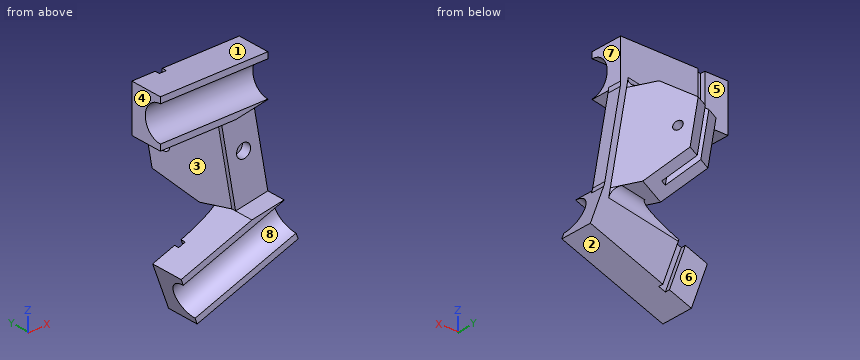
```python
from build123d import *

# Parameters (mm, degrees)
SKETCH2_W           = 58.42
SKETCH2_H           = 25.4
BOSS_EXTRUDE1_DEPTH = 17.78
CUT_EXTRUDE2_DEPTH  = 63.372388122
SKETCH6_W           = 3.81
SKETCH6_H           = 2.54
CUT_EXTRUDE3_DEPTH  = 25.4
CUT_EXTRUDE4_DEPTH  = 25.4
SKETCH8_W           = 17.78
SKETCH8_H           = 17.78
BOSS_EXTRUDE2_DEPTH = 25.4
SKETCH13_W          = 58.42
SKETCH13_H          = 9.398
CUT_EXTRUDE6_REACH  = 59.763
SKETCH15_W          = 25.4
SKETCH15_H          = 10.16
MIRROR14_START      = 9.31703521
MIRROR14_OUTLINE_W  = 7.62
MIRROR14_OUTLINE_H  = 25.4
MIRROR14_DEPTH      = 17.78
CUT_EXTRUDE7_DEPTH  = 25.4
BOSS_EXTRUDE3_DEPTH = 35.56
CUT_EXTRUDE8_REACH  = 128.018
CUT_EXTRUDE9_REACH  = 111.199
CUT_EXTRUDE10_REACH = 128.018
SKETCH25_R          = 2.4765
SKETCH26_R          = 3.81
CUT_EXTRUDE11_DEPTH = 5.08
FILLET1_R           = 15.24
FILLET2_R           = 5.08


with BuildPart() as part:
    # Sketch2 → Boss-Extrude1 (new body)
    with BuildSketch(Plane(origin=(0, 0, 0), x_dir=(1, 0, 0), z_dir=(0, 1, 0))):
        Rectangle(SKETCH2_W, SKETCH2_H)
    boss_extrude1 = extrude(amount=BOSS_EXTRUDE1_DEPTH)

    # Sketch4 → Cut-Extrude2 (cut, symmetric)
    with BuildSketch(Plane.ZY.offset(29.21)):
        with BuildLine():
            Line((-9.398, -66.725655712), (-9.398, 0))
            ThreePointArc((-9.398, 0), (0, 9.398), (9.398, 0))
            Line((9.398, 0), (9.398, -66.725655712))
            Line((9.398, -66.725655712), (9.398, -200.176967137))
            Line((9.398, -200.176967137), (-9.398, -200.176967137))
            Line((-9.398, -200.176967137), (-9.398, -66.725655712))
        make_face()
    cut_extrude2 = extrude(amount=CUT_EXTRUDE2_DEPTH, both=True, mode=Mode.SUBTRACT)

    # Sketch6 → Cut-Extrude3 (cut)
    with BuildSketch(Plane(origin=(0, 0, -12.7), x_dir=(-1, 0, 0), z_dir=(0, 0, -1))):
        with Locations((14.605, 16.51)):
            Rectangle(SKETCH6_W, SKETCH6_H)
    cut_extrude3 = extrude(amount=-CUT_EXTRUDE3_DEPTH, mode=Mode.SUBTRACT)

    # Sketch7 → Cut-Extrude4 (cut)
    with BuildSketch(Plane(origin=(0, 17.78, 0), x_dir=(1, 0, 0), z_dir=(0, 1, 0))):
        Polygon((11.700118151, 12.7), (29.21, 9.612535401), (29.21, 12.7), align=None)
    extrude(amount=-CUT_EXTRUDE4_DEPTH, mode=Mode.SUBTRACT)

    # Sketch8 → Boss-Extrude2 (add)
    with BuildSketch(Plane(origin=(2.524629641, 0, -14.317886186), x_dir=(-0.9848077530122094, 0, -0.17364817766692317), z_dir=(0.17364817766692317, 0, -0.9848077530122094))):
        with Locations((-18.20703521, 8.89)):
            Rectangle(SKETCH8_W, SKETCH8_H)
    extrude(amount=BOSS_EXTRUDE2_DEPTH)

    # Sketch13 → Cut-Revolve2 (revolve, cut)
    with BuildSketch(Plane.XZ):
        with Locations((0, 4.699)):
            Rectangle(SKETCH13_W, SKETCH13_H)
    revolve(axis=Axis((28.421300087, 0, 0), (-1, 0, 0)), mode=Mode.SUBTRACT)

    # Sketch15 → Cut-Extrude6 (cut, up to next)
    with BuildSketch(Plane(origin=(9.17548851, 0, 1.617886186), x_dir=(-0.17364817766692317, 0, 0.9848077530122095), z_dir=(-0.9848077530122095, 0, -0.17364817766692317)), mode=Mode.PRIVATE) as cut_extrude6_sk1:
        with Locations((-27.238762659, 5.08)):
            Rectangle(SKETCH15_W, SKETCH15_H)
    cut_extrude6_tool1 = extrude(cut_extrude6_sk1.sketch, amount=-CUT_EXTRUDE6_REACH, mode=Mode.PRIVATE) & part.part
    cut_extrude6 = cut_extrude6_tool1.solids().sort_by_distance((13.90545, 5.08, -25.207058))[0]
    add(cut_extrude6, mode=Mode.SUBTRACT)

    # Mirror14: read off the stored shape, not the designer's step
    # Mirror14 outline → Mirror14 (add)
    with BuildSketch(Plane(origin=(0, 0, 0), x_dir=(0, 1, 0), z_dir=(0.9848077530122094, 0, 0.17364817766692306)).offset(MIRROR14_START)):
        with Locations((13.97, -52.638762659)):
            Rectangle(MIRROR14_OUTLINE_W, MIRROR14_OUTLINE_H)
    extrude(amount=MIRROR14_DEPTH)

    # Mirror15: Boss-Extrude1 across plane
    add(boss_extrude1.mirror(Plane(origin=(6.935293354, 0, -39.332003112), x_dir=(0.9848077530122092, 0, 0.17364817766692314), z_dir=(0.17364817766692314, 0, -0.9848077530122094))))

    # Mirror16: Cut-Extrude2, Cut-Extrude3, Cut-Extrude6 across plane
    add(cut_extrude2.mirror(Plane(origin=(6.935293354, 0, -39.332003112), x_dir=(0.9848077530122092, 0, 0.17364817766692314), z_dir=(0.17364817766692314, 0, -0.9848077530122094))), mode=Mode.SUBTRACT)
    add(cut_extrude3.mirror(Plane(origin=(6.935293354, 0, -39.332003112), x_dir=(0.9848077530122092, 0, 0.17364817766692314), z_dir=(0.17364817766692314, 0, -0.9848077530122094))), mode=Mode.SUBTRACT)
    add(cut_extrude6.mirror(Plane(origin=(6.935293354, 0, -39.332003112), x_dir=(0.9848077530122092, 0, 0.17364817766692314), z_dir=(0.17364817766692314, 0, -0.9848077530122094))), mode=Mode.SUBTRACT)

    # Sketch21 → Cut-Extrude7 (cut, symmetric)
    with BuildSketch(Plane(origin=(6.935293354, 0, -39.332003112), x_dir=(-0.9848077530122094, 0, -0.17364817766692314), z_dir=(0.17364817766692314, 0, -0.9848077530122094))):
        Polygon((-23.83567521, 17.78), (-9.31703521, 12.495647198), (-9.31703521, 17.78), align=None)
    extrude(amount=CUT_EXTRUDE7_DEPTH, both=True, mode=Mode.SUBTRACT)

    # Sketch22 → Boss-Extrude3 (add)
    with BuildSketch(Plane(origin=(-2.881682913, 8.039496752, -0.508118447), x_dir=(-0.19346054761682988, -0.00733712504048707, 0.9810806200878379), z_dir=(-0.33682408883345943, 0.9396926207859106, -0.059391174613881166))):
        Polygon((-65.934673992, 27.071104434), (-15.146364467, 28.160882213), (-14.814917266, 12.714023803), (-65.603226791, 11.624246024), align=None)
    extrude(amount=BOSS_EXTRUDE3_DEPTH)

    # Sketch23 → Cut-Extrude8 (cut, up to next)
    with BuildSketch(Plane(origin=(26.355240658, 9.740503248, 4.647140011), x_dir=(0.3782029195796047, -0.8606292095735792, -0.3409984094540904), z_dir=(0.9254165783983268, 0.3420201433256624, 0.16317591116652866)), mode=Mode.PRIVATE) as cut_extrude8_sk1:
        Polygon((-19.269639975, 65.921874736), (4.43963551, 69.395008187), (-14.170689985, 77.55332817), align=None)
    cut_extrude8_tool1 = extrude(cut_extrude8_sk1.sketch, amount=-CUT_EXTRUDE8_REACH, mode=Mode.PRIVATE) & part.part
    # Sketch23 → Cut-Extrude8 (cut, up to next)
    with BuildSketch(Plane(origin=(26.355240658, 9.740503248, 4.647140011), x_dir=(0.3782029195796047, -0.8606292095735792, -0.3409984094540904), z_dir=(0.9254165783983268, 0.3420201433256624, 0.16317591116652866)), mode=Mode.PRIVATE) as cut_extrude8_sk2:
        Polygon((-15.956164448, 22.869194448), (-34.566489944, 31.027514432), (-29.467539954, 42.658967866), align=None)
    cut_extrude8_tool2 = extrude(cut_extrude8_sk2.sketch, amount=-CUT_EXTRUDE8_REACH, mode=Mode.PRIVATE) & part.part
    add(cut_extrude8_tool1.solids().sort_by_distance((24.388361, 44.830618, -57.747753))[0], mode=Mode.SUBTRACT)
    add(cut_extrude8_tool2.solids().sort_by_distance((17.037255, 44.830618, -16.057558))[0], mode=Mode.SUBTRACT)

    # Cut-Extrude9: up to this plane
    cut_extrude9_end = Plane(origin=(-45.924606639, 26.595398182, -61.548547649), z_dir=(0.031263049894144905, -0.49803609294534235, 0.8665925639163162))
    # Sketch24 → Cut-Extrude9 (cut, up to the surface)
    with BuildSketch(Plane(origin=(2.524629641, 0, -14.317886186), x_dir=(-0.9848077530122095, 0, -0.1736481776669232), z_dir=(0.1736481776669232, 0, -0.9848077530122095)), mode=Mode.PRIVATE) as cut_extrude9_sk1:
        Polygon((-8.170546151, 33.702451643), (-11.082465645, 34.762303663), (-5.87007866, 49.083219204), (-2.958159167, 48.023367184), align=None)
    cut_extrude9_tool1 = split(extrude(cut_extrude9_sk1.sketch, amount=CUT_EXTRUDE9_REACH, mode=Mode.PRIVATE), bisect_by=cut_extrude9_end, keep=Keep.BOTH, mode=Mode.PRIVATE)
    add(cut_extrude9_tool1.solids().sort_by_distance((9.438288, 41.392835, -13.098822))[0], mode=Mode.SUBTRACT)

    # Cut-Extrude10: up to this face of the body (flat: up to its plane)
    cut_extrude10_end = Plane(part.part.faces().sort_by_distance((10.739934643, 27.479568088, -38.661142201))[0])
    # Sketch25 → Cut-Extrude10 (cut, up to the picked face)
    with BuildSketch(Plane(origin=(26.355240658, 9.740503248, 4.647140011), x_dir=(0.3782029195796047, -0.8606292095735792, -0.3409984094540904), z_dir=(0.9254165783983268, 0.3420201433256624, 0.16317591116652866)), mode=Mode.PRIVATE) as cut_extrude10_sk1:
        with Locations(Location((-17.389717904, 51.231051307, 0), (0, 0, 159.779686777))):
            Circle(SKETCH25_R)
    cut_extrude10_tool1 = split(extrude(cut_extrude10_sk1.sketch, amount=-CUT_EXTRUDE10_REACH, mode=Mode.PRIVATE), bisect_by=cut_extrude10_end, keep=Keep.BOTH, mode=Mode.PRIVATE)
    add(cut_extrude10_tool1.solids().sort_by(Axis((20.997986, 44.035012, -36.852371), (-0.9254165783983268, -0.3420201433256624, -0.16317591116652866)))[0], mode=Mode.SUBTRACT)

    # Sketch26 → Cut-Extrude11 (cut)
    with BuildSketch(Plane.XZ.offset(-10.16)):
        with Locations(Location((24.865722788, -36.170384627, 0), (0, 0, 270))):
            Circle(SKETCH26_R)
    extrude(amount=-CUT_EXTRUDE11_DEPTH, mode=Mode.SUBTRACT)

    # Fillet1
    fillet1_edges = [part.edges().sort_by_distance(p)[0] for p in [
        (29.21, 13.97, -9.612535401),
        (38.031327425, 13.97, -59.640769254),
    ]]
    fillet(fillet1_edges, radius=FILLET1_R)

    # Fillet2
    # the kernel refuses this fillet: 5.08 mm, written as the material it adds along each edge
    with BuildSketch(Plane(origin=(-16.999729813, 17.78, -69.344229422), x_dir=(0.17364817766692311, 0, -0.9848077530122094), z_dir=(0.9848077530122094, 0, 0.17364817766692314))) as fillet2_piece_1_section:
        with BuildLine():
            CenterArc((FILLET2_R, FILLET2_R), FILLET2_R, 180, 90)
            Line((0, FILLET2_R), (0, 0))
            Line((0, 0), (FILLET2_R, 0))
        make_face()
    fillet2_piece_1 = extrude(amount=65.31864, mode=Mode.PRIVATE)
    fillet2_piece_1 = split(fillet2_piece_1, bisect_by=Plane(origin=(28.757814695, 34.691304915, -61.275939754), z_dir=(-0.925416578398327, -0.34202014332566266, -0.16317591116652855)), keep=Keep.TOP, mode=Mode.PRIVATE)
    fillet2_piece_1 = split(fillet2_piece_1, bisect_by=Plane(origin=(-4.669969149, 17.78, -64.856563545), z_dir=(0.9396926207859135, 0, 0.342020143325655)), keep=Keep.TOP, mode=Mode.PRIVATE)
    fillet2_piece_1 = split(fillet2_piece_1, bisect_by=Plane(origin=(-14.73692606, 17.78, -75.561231638), z_dir=(0.342020143325655, 0, -0.9396926207859134)), keep=Keep.TOP, mode=Mode.PRIVATE)
    add(fillet2_piece_1)
    with BuildSketch(Plane(origin=(-25.821057238, 17.78, -19.315995569), x_dir=(-0.17364817766692314, 0, 0.9848077530122094), z_dir=(0.9848077530122094, 0, 0.17364817766692314))) as fillet2_piece_2_section:
        with BuildLine():
            CenterArc((FILLET2_R, -FILLET2_R), FILLET2_R, 90, 90)
            Line((0, -FILLET2_R), (0, 0))
            Line((0, 0), (FILLET2_R, 0))
        make_face()
    fillet2_piece_2 = extrude(amount=65.31864, mode=Mode.PRIVATE)
    fillet2_piece_2 = split(fillet2_piece_2, bisect_by=Plane(origin=(-12.7, 17.78, -19.315995569), z_dir=(1, 0, 0)), keep=Keep.TOP, mode=Mode.PRIVATE)
    fillet2_piece_2 = split(fillet2_piece_2, bisect_by=Plane(origin=(-25.821057238, 17.78, -12.7), z_dir=(0, 0, 1)), keep=Keep.TOP, mode=Mode.PRIVATE)
    fillet2_piece_2 = split(fillet2_piece_2, bisect_by=Plane(origin=(19.93648727, 34.691304915, -11.247705901), z_dir=(-0.925416578398327, -0.34202014332566266, -0.16317591116652855)), keep=Keep.TOP, mode=Mode.PRIVATE)
    add(fillet2_piece_2)


solid = part.part
```
Design review of the part built by this model. Coordinates are the model's own, in mm. Face numbers are marked on the shaded views. A direction names the side the tool comes from. Give positions to 0.01 mm unless a question says otherwise; leave off trailing zeros. Write each loop counter-clockwise with the first axis right and the second up, starting at its lowest first coordinate (ties: lowest second). Pieces come first, ordered by that corner, then holes.
(1) Add section C-C (z = -28.5). Give the boundary of the cut face in (x, y), and give its area (3 significant figures).
Checked values:
outline: (2.14, 45.91) - (14.49, 12.5) - (14.49, 10.16) - (32.54, 10.16) - (32.54, 17.78) - (29.23, 17.78) - (16.88, 51.2) - (10.99, 49.08) - (16.28, 34.76) - (13.32, 33.7) - (8.03, 48.02) - close
area: 609 mm2
(2) Add section B-B (z = 0). Give the boundary of the cut face in (x, y), and give its area (3 significant figures).
Checked values:
outline: (-29.21, 9.4) - (29.21, 9.4) - (29.21, 17.78) - (-12.7, 17.78) - (-12.7, 15.24) - (-16.51, 15.24) - (-16.51, 17.78) - (-29.21, 17.78) - close
area: 480 mm2
(3) Mouldability with a two-part tool opening along Z and no side actions: class the marked faces 1, 2, 3 and 4 as +Z half, -Z half, draft (parallel to the pull), parting line (faces both ways), or undercut.
Checked values:
face 1: +Z half
face 2: -Z half
face 3: undercut
face 4: draft
(4) Add section A-A (y = 3). Give the boundary of the cut face in (x, z).
Checked values:
outline: (-29.21, -12.7) - (11.7, -12.7) - (29.21, -9.61) - (29.21, -8.91) - (-29.21, -8.91) - close; (-29.21, 8.91) - (29.21, 8.91) - (29.21, 12.7) - (-29.21, 12.7) - close; (-17.92, -76.72) - (-16.62, -80.29) - (38.27, -60.3) - (38.03, -59.64) - (20.52, -62.73) - close; (-10.53, -97.02) - (-9.23, -100.59) - (45.66, -80.61) - (44.37, -77.04) - close
(5) Tool access review of the marked faces 5, 6, 7 and 8: name each direction out of +Z, -Z, +X, -X, +Y, -Y from which nothing blocks a thin tool from reaching the whole face with its end or side.
Checked values:
face 5: +Z, -Z, -X, +Y
face 6: -Z, +X, -X, +Y
face 7: +Z, +X, +Y, -Y
face 8: -Y
(6) Clearance check with flat-ended pins moving along their axes: pin 1 Ø3.5 at (x, z) = (-2.5, -80.5) entering from +Y; pin 2 Ø6 at (y, z) = (28.5, -10.5) entering from +X; pin 3 Ø2 at (x, z) = (3, -79.5) entering from -Y; pin 4 Ø18.5 at (x, y) = (-17.5, 6) entering from -Z. State where each tip first meets the part, or that it passes through.
Checked values:
pin 1: stops at y = 17.78
pin 2: stops at x = 23.32
pin 3: stops at y = 8.54
pin 4: stops at z = -100.59
(7) Wall thickness on line 1 along Z through (x, y) = (5, 2); line 2 along Z through (x, y) = (35, 7); line 3 along X through (y, z) = (12, -39.5): over which ranges is each line inside the solid? List them lowest first.
Checked values:
line 1: z = -95.41 to -91.66, -72.12 to -68.38, -12.7 to -9.18, 9.18 to 12.7
line 2: z = -84.49 to -77.65, -64.3 to -60.18
line 3: x = 16.43 to 23.01, 26.72 to 34.48
